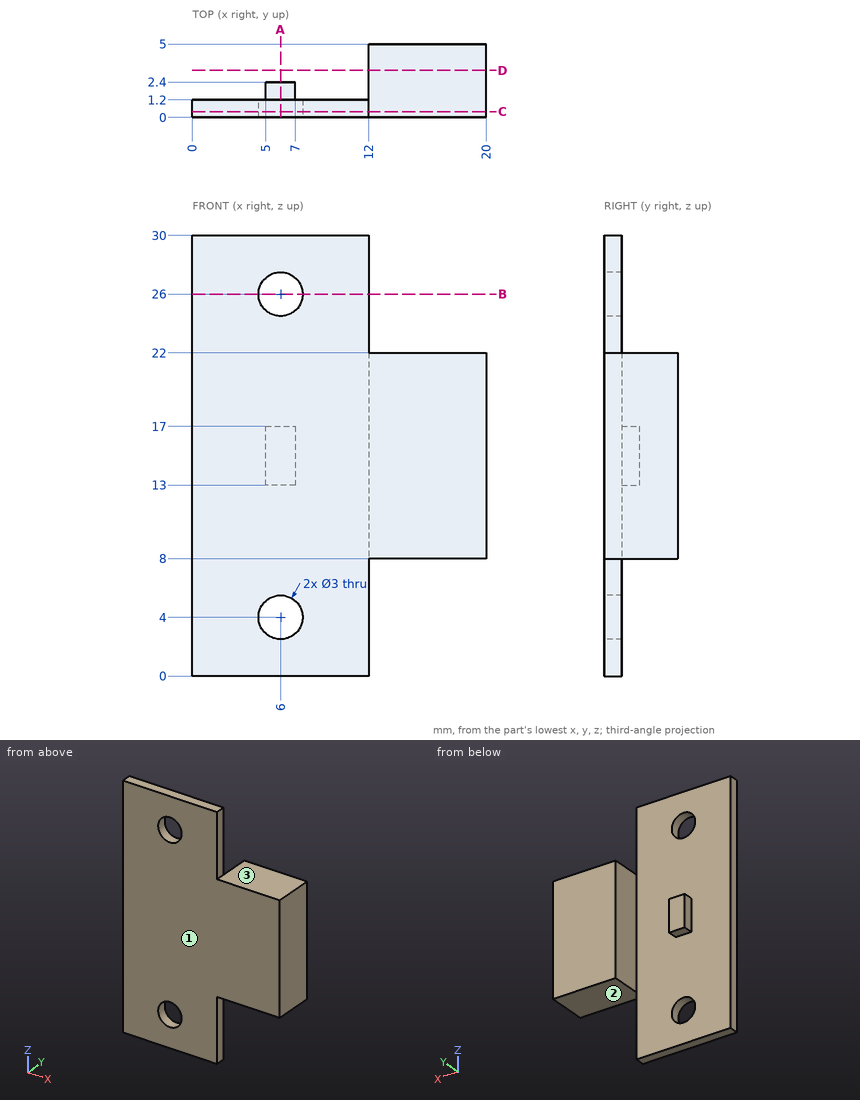
Drawing for the job (mm, zero at the part's lowest x, y, z). A direction names the side the tool comes from. Give positions to 0.01 mm unless a question says otherwise; leave off trailing zeros. Loops run counter-clockwise (first coordinate to the right, second up) from the corner with the lowest first, then second, coordinate; pieces in that order, holes last. Notation, with made-up numbers: (-0.75, -10) - (48.25, -10) arc R28 cw to (48.25, 11) - close; hole circle Ø6 at (88, 78). An arc over 180 degrees is marked (long way). Write item = value, one per line. Start each with the question number.
1) Tool access for the marked faces 1, 2 and 3: list every direction of +Z, -Z, +X, -X, +Y, -Y with a clear straight run to the whole face (end or side of a thin tool).
2) Probe probe 1 along Z at (x, y) = (6, 0.75); probe 2 along Y at (x, z) = (4.5, 13); probe 3 along Z at (x, y) = (17, 3.1). List the from-to ranges inside material, lowest first. Write a range as from..to.
3) Band-saw the part on C-C on y = 0.4. Give the cut face in (x, z).
4) Band-saw the part on B-B on z = 26. Give the cut face in (x, y).
5) Band-saw the part on A-A on x = 6. Give the cut face in (y, z), plus the area to 3 significant figures.
6) Band-saw the part on D-D on y = 3.2. Give the cut face in (x, z), plus the area to 3 significant figures.
7) Drop flat-ended pins along their axis: pin 1 Ø1.6 at (x, z) = (6, 14) entering from +Y; pin 2 Ø1 at (y, z) = (2.5, 19) entering from -X; pin 3 Ø2.5 at (x, z) = (6, 26) entering from +Y; pin 4 Ø3 at (x, y) = (15.5, 4) entering from +Z. Give the stop position or say it passes through.
Final values:
q1.face_1 = +Z, -Z, +X, -X, -Y
q1.face_2 = -Z, +X, +Y, -Y
q1.face_3 = +Z, +X, +Y, -Y
q2.probe_1 = 0..2.5, 5.5..24.5, 27.5..30
q2.probe_2 = 0..1.2
q2.probe_3 = 8..22
q3.outline = (0, 0) - (12, 0) - (12, 8) - (20, 8) - (20, 22) - (12, 22) - (12, 30) - (0, 30) - close; hole circle Ø3 at (6, 4); hole circle Ø3 at (6, 26)
q4.outline = (0, 0) - (4.5, 0) - (4.5, 1.2) - (0, 1.2) - close; (7.5, 0) - (12, 0) - (12, 1.2) - (7.5, 1.2) - close
q5.outline = (0, 0) - (1.2, 0) - (1.2, 2.5) - (0, 2.5) - close; (0, 5.5) - (1.2, 5.5) - (1.2, 13) - (2.4, 13) - (2.4, 17) - (1.2, 17) - (1.2, 24.5) - (0, 24.5) - close; (0, 27.5) - (1.2, 27.5) - (1.2, 30) - (0, 30) - close
q5.area = 33.6 mm²
q6.outline = (12, 8) - (20, 8) - (20, 22) - (12, 22) - close
q6.area = 112 mm²
q7.pin_1 = 2.4
q7.pin_2 = 12
q7.pin_3 = through
q7.pin_4 = 22
